from build123d import *

# Parameters (mm, degrees)
F0_W     = 6.35
F0_H     = 6.35
F1_DEPTH = 6.35


with BuildPart() as f1:
    # F0 (on Top) → F1 (new body)
    with BuildSketch(Plane.XY):
        Polygon((9.525, 0), (0, 0), (0, -9.525), (0, -15.875), (0, -25.4), (9.525, -25.4), (15.875, -25.4), (25.4, -25.4), (25.4, -15.875), (25.4, -9.525), (25.4, 0), (15.875, 0), align=None)
        with Locations((12.7, 3.175)):
            Rectangle(F0_W, F0_H)
        with Locations((-3.175, -12.7)):
            Rectangle(F0_W, F0_H)
        with Locations((28.575, -12.7)):
            Rectangle(F0_W, F0_H)
        with Locations((12.7, -28.575)):
            Rectangle(F0_W, F0_H)
    extrude(amount=F1_DEPTH)


solid = f1.part
Design review of the part built by this model. Coordinates are the model's own, in mm. A direction names the side the tool comes from. Give positions to 0.01 mm unless a question says otherwise; leave off trailing zeros. Loops run counter-clockwise (first coordinate to the right, second up) from the corner with the lowest first, then second, coordinate; pieces in that order, holes last. Notation, with made-up numbers: (-37.75, 74.5) -> (-17.75, 74.5) arc R22 cw to (-17.75, 96.5) -> close; hole circle Ø7 at (-15.75, 45). An arc over 180 degrees is marked (long way). One line per question, with ' | ' between items. Start each with the question number.
(1) For faces 1 (the face through (25.4, -5, 3)), 2 (the face through (-3, -9.525, 3)), 3 (the face through (5, -25.4, 3)), 4 (the face through (29, -15.875, 3)), 5 (the face through (-6.35, -13, 3)), list the 3-axis set-ups (+Z, -Z, +X, -X, +Y, -Y) from which the entire face can be reached by the end or side of a thin tool; tool diameter is ignored.
(2) For line 1 (Y direction, x = 19.5, z = 3); line 2 (X direction, y = -4.5, z = 1.75); line 3 (Y direction, x = -4, z = 2.25) (3 decimals), list the stretches that pass through material, from the lowest coordinate up.
(3) Insertion check: P1, Ø3, axis at x = 28.5, z = 3.5, coming from the +Y side (3 decimals); P2, Ø10, axis at x = 4.5, y = -27.5, coming from the -Z side; P3, Ø1.9, axis at y = -27.5, z = 3.5, coming from the -X side (3 decimals); P4, Ø1.9, axis at x = 6.5, z = 4.5, coming from the -Y side. Each pin has a flat end and moves straight along its axis. Give the tip position at first contact, or say it passes through.
(4) We need section A-A (z = 3.5). State the section outline as (x, y) points (3 decimals).
(5) We need section B-B (x = 29.5). State the section outline as (y, z) points (3 decimals).
(6) We need section C-C (x = 23.5). State the section outline as (y, z) points, and give its area (3 significant figures).
The answers:
1) face 1: +Z, -Z, +X, +Y | face 2: +Z, -Z, -X, +Y | face 3: +Z, -Z, -X, -Y | face 4: +Z, -Z, +X, -Y | face 5: +Z, -Z, -X, +Y, -Y
2) line 1: y = -25.4 to 0 | line 2: x = 0 to 25.4 | line 3: y = -15.875 to -9.525
3) P1: stops at y = -9.525 | P2: stops at z = 0 | P3: stops at x = 9.525 | P4: stops at y = -25.4
4) outline: (-6.35, -15.875) -> (0, -15.875) -> (0, -25.4) -> (9.525, -25.4) -> (9.525, -31.75) -> (15.875, -31.75) -> (15.875, -25.4) -> (25.4, -25.4) -> (25.4, -15.875) -> (31.75, -15.875) -> (31.75, -9.525) -> (25.4, -9.525) -> (25.4, 0) -> (15.875, 0) -> (15.875, 6.35) -> (9.525, 6.35) -> (9.525, 0) -> (0, 0) -> (0, -9.525) -> (-6.35, -9.525) -> close
5) outline: (-15.875, 0) -> (-9.525, 0) -> (-9.525, 6.35) -> (-15.875, 6.35) -> close
6) outline: (-25.4, 0) -> (0, 0) -> (0, 6.35) -> (-25.4, 6.35) -> close | area: 161 mm^2
